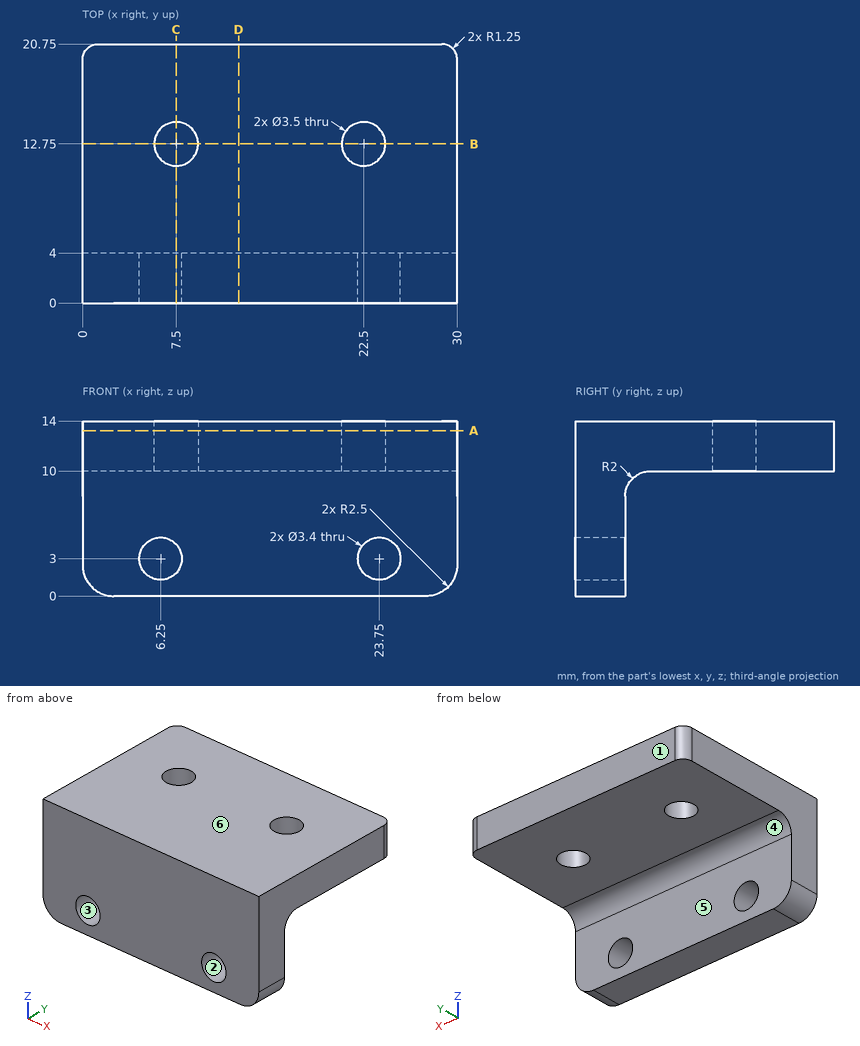
Check sheet for the drawn part. Datum: minimum x, y, z corner. Units: mm. A direction names the side the tool comes from. Give positions to 0.01 mm unless a question says otherwise; leave off trailing zeros. Loops run counter-clockwise (first coordinate to the right, second up) from the corner with the lowest first, then second, coordinate; pieces in that order, holes last.
1) Thickness scan on line 1 along X through (y, z) = (0.9, 3); line 2 along Z through (x, y) = (23.75, 1.45); line 3 along Z through (x, y) = (21.75, 7). Record the ranges inside material, lowest first.
2) Sectioned sample at C-C, the plane x = 7.5. Enter the section's corners in (y, z), then the cut area to 3 significant figures.
3) Sectioned sample at B-B, the plane y = 12.75. Enter the section's corners in (x, z).
4) Set-up check for the marked faces 5 and 6: record each of +Z, -Z, +X, -X, +Y, -Y from which the full face is reachable in a straight line by a thin tool's end or side.
5) Sectioned sample at D-D, the plane x = 12.5. Enter the section's corners in (y, z).
6) Draft check along Z on the marked faces 1, 2, 3 and 4. Enter one of: pulls with the +Z half, pulls with the -Z half, needs draft (parallel to the pull), parting line crosses it, or undercut.
7) Depth check by flat-ended pin: pin 1 Ø12 at (x, y) = (9.5, 13) entering from -Z; pin 2 Ø4.5 at (x, z) = (6.25, 3) entering from +Y; pin 3 Ø2 at (x, y) = (19.5, 6) entering from -Z; pin 4 Ø8 at (y, z) = (18.5, 5) entering from +X. Enter the tip coordinate at first touch or a pass-through.
8) Sectioned sample at A-A, the plane z = 13.25. Enter the section's corners in (x, y).
Answers:
1. line 1: x = 0 to 4.55, 7.95 to 22.05, 25.45 to 30
1. line 2: z = 0 to 1.3, 4.7 to 14
1. line 3: z = 10 to 14
2. outline: (0, 0) - (4, 0) - (4, 1.85) - (0, 1.85) - close; (0, 4.15) - (4, 4.15) - (4, 8) arc R2 cw to (6, 10) - (11, 10) - (11, 14) - (0, 14) - close; (14.5, 10) - (20.75, 10) - (20.75, 14) - (14.5, 14) - close
2. area: 101 mm2
3. outline: (0, 10) - (5.75, 10) - (5.75, 14) - (0, 14) - close; (9.25, 10) - (20.75, 10) - (20.75, 14) - (9.25, 14) - close; (24.25, 10) - (30, 10) - (30, 14) - (24.25, 14) - close
4. face 5: -Z, +X, -X, +Y
4. face 6: +Z, +X, -X, +Y, -Y
5. outline: (0, 0) - (4, 0) - (4, 8) arc R2 cw to (6, 10) - (20.75, 10) - (20.75, 14) - (0, 14) - close
6. face 1: needs draft
6. face 2: undercut
6. face 3: undercut
6. face 4: pulls with the -Z half
7. pin 1: stops at z = 10
7. pin 2: stops at y = 4
7. pin 3: stops at z = 9.73
7. pin 4: passes through
8. outline: (0, 0) - (30, 0) - (30, 19.5) arc R1.25 ccw to (28.75, 20.75) - (1.25, 20.75) arc R1.25 ccw to (0, 19.5) - close; hole circle Ø3.5 at (7.5, 12.75); hole circle Ø3.5 at (22.5, 12.75)
